```python
from build123d import *

# Parameters (mm, degrees)
SKETCH1_R           = 5
SKETCH1_R_2         = 3.25
BOSS_EXTRUDE1_DEPTH = 3
FILLET1_R           = 2


with BuildPart() as part:
    # Sketch1 → Boss-Extrude1 (new body, symmetric)
    with BuildSketch(Plane(origin=(0, 0, 0), x_dir=(1, 0, 0), z_dir=(0, 1, 0))):
        with BuildLine():
            Line((-5, 5), (-5, 0))
            ThreePointArc((-5, 0), (-3.535533906, 3.535533906), (0, 5))
            Line((0, 5), (-5, 5))
        make_face()
        Circle(SKETCH1_R)
        Circle(SKETCH1_R_2, mode=Mode.SUBTRACT)
        with BuildLine():
            ThreePointArc((0, 5), (3.535533906, 3.535533906), (5, 0))
            Line((5, 0), (5, 5))
            Line((5, 5), (0, 5))
        make_face()
        with BuildLine():
            ThreePointArc((5, 0), (3.535533906, -3.535533906), (0, -5))
            Line((0, -5), (5, -5))
            Line((5, -5), (5, 0))
        make_face()
        with BuildLine():
            Line((-5, 0), (-5, -5))
            Line((-5, -5), (0, -5))
            ThreePointArc((0, -5), (-3.535533906, -3.535533906), (-5, 0))
        make_face()
    extrude(amount=BOSS_EXTRUDE1_DEPTH, both=True)

    # Fillet1
    fillet1_edges = [part.edges().sort_by_distance(p)[0] for p in [
        (-5, 0, -5),
        (5, 0, -5),
        (5, 0, 5),
        (-5, 0, 5),
    ]]
    fillet(fillet1_edges, radius=FILLET1_R)


solid = part.part
```
Read the model definition and answer for the solid it produces. Units are mm, in the model's axes. Coordinates: 2 decimals unless noted, no trailing zeros. Write each loop counter-clockwise with the first axis right and the second up, starting at its lowest first coordinate (ties: lowest second). Pieces come first, ordered by that corner, then holes. Notation, with made-up numbers: (-3.5, -1.5) -> (1.5, -1.5) arc R31 ccw to (1.5, 32.5) -> close; hole circle Ø9 at (86.5, -25). An arc over 180 degrees is marked (long way). Answer as a JSON object with one key per item and string values.
Q1. Determine the mould class of faces 1 (the flat face through (-5, 0, 0)), 2 (the cylindrical face through (-2.579, -0.042, 1.978)), 3 (the cylindrical face through (4.43, 0.04, 4.4)), 4 (the flat face through (0, 0, -5)) for opening direction X: pulls with the +X half, pulls with the -X half, needs draft (parallel to the pull), parting line crosses it, or undercut.
The answers:
{"face 1": "pulls with the -X half", "face 2": "undercut", "face 3": "pulls with the +X half", "face 4": "needs draft"}
Q2. Consider line 1 (Z direction, x = 0, y = 1.3); line 2 (X direction, y = -2.65, z = 1.5). Determine where each line is inside the solid, lowest interval first. Write a range as [from, to].
The answers:
{"line 1": "z = [-5, -3.25], [3.25, 5]", "line 2": "x = [-5, -2.88], [2.88, 5]"}
Q3. The part is cut by section D-D on z = 4.25. Give the vertices of the cut face in (x, y), then the cut area to 3 significant figures.
The answers:
{"outline": "(-4.56, -3) -> (4.56, -3) -> (4.56, 3) -> (-4.56, 3) -> close", "area": "54.7 mm2"}
Q4. The part is cut by section B-B on y = -1.15. Give the vertices of the cut face in (x, z), then the cut area to 3 significant figures.
The answers:
{"outline": "(-5, -3) arc R2 ccw to (-3, -5) -> (3, -5) arc R2 ccw to (5, -3) -> (5, 3) arc R2 ccw to (3, 5) -> (-3, 5) arc R2 ccw to (-5, 3) -> close; hole circle Ø6.5 at (0, 0)", "area": "63.4 mm2"}
Q5. A flat-ended cylindrical pin translates along its axis: pin 1 Ø6 at (x, z) = (0, 0) entering from -Y. Find the tip coordinate at first contact, or state that the pin passes through.
The answers:
{"pin 1": "passes through"}
Q6. The part is cut by section C-C on z = 0. Give the vertices of the cut face in (x, y), then the cut area to 3 significant figures.
The answers:
{"outline": "(-5, -3) -> (-3.25, -3) -> (-3.25, 3) -> (-5, 3) -> close; (3.25, -3) -> (5, -3) -> (5, 3) -> (3.25, 3) -> close", "area": "21.0 mm2"}
Q7. The part is cut by section A-A on x = 0. Give the vertices of the cut face in (y, z), then the cut area to 3 significant figures.
The answers:
{"outline": "(-3, -5) -> (3, -5) -> (3, -3.25) -> (-3, -3.25) -> close; (-3, 3.25) -> (3, 3.25) -> (3, 5) -> (-3, 5) -> close", "area": "21.0 mm2"}
